Verification items for the finished model (mm, model axes). Coordinates: 2 decimals unless noted, no trailing zeros. Write each loop counter-clockwise with the first axis right and the second up, starting at its lowest first coordinate (ties: lowest second). Pieces come first, ordered by that corner, then holes.
Autodesk Inventor part; units mm, degrees
ref_plane "YZ Plane" through (0, 0, 0) normal (1, 0, 0) x (0, 1, 0)
ref_plane "XZ Plane" through (0, 0, 0) normal (0, 1, 0) x (-1, 0, 0)
ref_plane "XY Plane" through (0, 0, 0) normal (0, 0, 1) x (1, 0, 0)
sketch "Sketch1" plane through (0, 0, 0) normal (0, 0, 1) x (1, 0, 0)
  line L0 (-25.8084, 16.7799) -> (37.6916, 16.7799)
  line L1 (37.6916, 16.7799) -> (37.6916, -14.9701)
  line L2 (37.6916, -14.9701) -> (-25.8084, -14.9701)
  line L3 (-25.8084, -14.9701) -> (-25.8084, 16.7799)
  point P0 (0, 0)
  dimension "d0" = 31.75
  dimension "d1" = 63.5
extrude "Extrusion1" add sketch "Sketch1" along normal blind 1.5875
sketch "Sketch2" plane through (0, 0, 1.5875) normal (0, 0, 1) x (1, 0, 0)
  line L0 (37.6916, 16.7799) -> (37.6916, -14.9701)
  line L1 (-25.8084, 16.7799) -> (37.6916, 16.7799)
  line L2 (-25.8084, -14.9701) -> (-25.8084, 16.7799)
  line L3 (37.6916, -14.9701) -> (-25.8084, -14.9701)
  circle A0 centre (33.813, 12.9013) radius 1.5875
  circle A1 centre (33.813, -11.0915) radius 1.5875
  circle A2 centre (33.813, 2.4924) radius 0.7937
  circle A3 centre (33.813, 0.9049) radius 0.7937
  circle A4 centre (33.813, -0.6826) radius 0.7937
  line L4 (33.813, -14.9701) -> (33.813, 16.7799) construction
  line L5 (33.813, 2.4924) -> (33.813, 0.9049) construction
  line L6 (33.813, 0.9049) -> (33.813, -0.6826) construction
  line L7 (33.813, 12.9013) -> (33.813, 2.4924) construction
  line L8 (33.813, -11.0915) -> (33.813, -0.6826) construction
  circle A5 centre (-21.9298, 12.9013) radius 1.5875
  circle A6 centre (-21.9298, -11.0915) radius 1.5875
  line L9 (-21.9298, 16.7799) -> (-21.9298, -14.9701) construction
  line L10 (-25.8084, -11.0915) -> (37.6916, -11.0915) construction
  circle A7 centre (-15.5798, 12.9013) radius 1.5875
  circle A8 centre (-15.5798, -11.0915) radius 1.5875
  circle A9 centre (-2.8798, 12.9013) radius 1.5875
  circle A10 centre (-2.8798, -11.0915) radius 1.5875
  circle A11 centre (9.8202, 12.9013) radius 1.5875
  circle A12 centre (9.8202, -11.0915) radius 1.5875
  point P0 (0, 0)
  dimension "d4" = 3.8786
  dimension "d5" = 3.8786
  dimension "d6" = 3.8786
  dimension "d7" = 3.175
  dimension "d8" = 1.5875
  dimension "d9" = 3.175
  dimension "d10" = 3.8786
  dimension "d11" = 3.8786
  dimension "d14" = 6.35
  dimension "d21" = 12.7
  dimension "d28" = 12.7
extrude "Extrusion2" add sketch "Sketch2" along normal blind 0.254 contours A0 | A1 | A2 | A4 | A3 | A5 | A6 | A7 | A8 | A9 | A10 | A11 | A12
sketch "Sketch3" plane through (33.813, 12.9013, 1.8415) normal (0, 0, 1) x (1, 0, 0)
  circle A0 centre (0, 0) radius 1.5875 construction
sketch "Sketch4" plane through (33.813, -11.0915, 1.8415) normal (0, 0, 1) x (1, 0, 0)
  circle A0 centre (0, 0) radius 1.5875 construction
sketch "Sketch5" plane through (9.8202, 12.9013, 1.8415) normal (0, 0, 1) x (1, 0, 0)
  circle A0 centre (0, 0) radius 1.5875 construction
sketch "Sketch6" plane through (9.8202, -11.0915, 1.8415) normal (0, 0, 1) x (1, 0, 0)
  circle A0 centre (0, 0) radius 1.5875 construction
sketch "Sketch7" plane through (-2.8798, 12.9013, 1.8415) normal (0, 0, 1) x (1, 0, 0)
  circle A0 centre (0, 0) radius 1.5875 construction
sketch "Sketch8" plane through (-2.8798, -11.0915, 1.8415) normal (0, 0, 1) x (1, 0, 0)
  circle A0 centre (0, 0) radius 1.5875 construction
sketch "Sketch9" plane through (-15.5798, 12.9013, 1.8415) normal (0, 0, 1) x (1, 0, 0)
  circle A0 centre (0, 0) radius 1.5875 construction
sketch "Sketch10" plane through (-15.5798, -11.0915, 1.8415) normal (0, 0, 1) x (1, 0, 0)
  circle A0 centre (0, 0) radius 1.5875 construction
sketch "Sketch11" plane through (-21.9298, 12.9013, 1.8415) normal (0, 0, 1) x (1, 0, 0)
  circle A0 centre (0, 0) radius 1.5875 construction
sketch "Sketch12" plane through (-21.9298, -11.0915, 1.8415) normal (0, 0, 1) x (1, 0, 0)
  circle A0 centre (0, 0) radius 1.5875 construction
sketch "Sketch13" plane through (33.813, -0.6826, 1.8415) normal (0, 0, 1) x (1, 0, 0)
  circle A0 centre (0, 0) radius 0.7937 construction
  point P0 (0, 0.7937)
sketch "Sketch14" plane through (0, 0, 1.8415) normal (0, 0, 1) x (1, 0, 0)
  arc A0 (33.813, 0.1112) -> (33.813, 1.6987) centre (33.813, 0.9049) ccw construction
sketch "Sketch15" plane through (33.813, 2.4924, 1.8415) normal (0, 0, 1) x (1, 0, 0)
  circle A0 centre (0, 0) radius 0.7937 construction
  point P0 (0, -0.7937)
equation "\"d5\" = d4"
equation "\"d6\" = d4"
equation "\"d10\" = d4"
equation "\"d11\" = d4"
properties part number "PDU"
1. Material ranges on L1, parallel to X at y = 13, z = 1.7; L2, parallel to Z at x = -10.5, y = 10.5, recorded low to high.
2. Sectioned sample at B-B, the plane x = 9.5. Record the boundary of the cut face in (y, z).
3. Sectioned sample at A-A, the plane y = 4. Record the boundary of the cut face in (x, z), and give its area (3 significant figures).
4. Sectioned sample at C-C, the plane x = 18. Record the boundary of the cut face in (y, z), and give its area (3 significant figures).
5. Gauge pin test, flat end, axial feed: P1, Ø8, axis at x = 18.5, y = -10, coming from the +Z side. Record the tip position at first contact, or that the pin passes through.
Outcome:
1. L1: x = -23.51 to -20.35, -17.16 to -14, -4.46 to -1.3, 8.24 to 11.4, 32.23 to 35.4
1. L2: z = 0 to 1.59
2. outline: (-14.97, 0) - (16.78, 0) - (16.78, 1.59) - (14.46, 1.59) - (14.46, 1.84) - (11.35, 1.84) - (11.35, 1.59) - (-9.54, 1.59) - (-9.54, 1.84) - (-12.65, 1.84) - (-12.65, 1.59) - (-14.97, 1.59) - close
3. outline: (-25.81, 0) - (37.69, 0) - (37.69, 1.59) - (-25.81, 1.59) - close
3. area: 101 mm2
4. outline: (-14.97, 0) - (16.78, 0) - (16.78, 1.59) - (-14.97, 1.59) - close
4. area: 50.4 mm2
5. P1: stops at z = 1.59
